For this review, take the finished solid that the model builds, in its own axes (mm). Give positions to 0.01 mm unless a question says otherwise; leave off trailing zeros. Loops run counter-clockwise (first coordinate to the right, second up) from the corner with the lowest first, then second, coordinate; pieces in that order, holes last. Notation, with made-up numbers: (51, 8.25) - (102, 8.25) arc R22 ccw to (102, 39.25) - close; hole circle Ø9 at (-17.5, 82.25). An arc over 180 degrees is marked (long way). Use CSV: the item, a comma, the result in double quotes. Start each with the question number.
1. Mouldability with a two-part tool opening along X and no side actions: class faces 1 (the cylindrical face through (2.71, 0.7, -62.203)), 2 (the flat face through (-50, -1, -222)), 3 (the flat face through (50, -1, -222)) as pulls with the +X half, pulls with the -X half, needs draft (parallel to the pull), parting line crosses it, or undercut.
2. Take a section at B-B on z = -50. Give the boundary of the cut face in (x, y), plus the area to 3 significant figures.
3. Wall thickness on line 1 (Z direction, x = 0, y = -3); line 2 (Z direction, x = -3.5, y = -14): over which ranges is each line inside the solid? List them lowest first.
4. For pin 1 (15 mm diameter, centred on x = 0, z = -50, fed in from +Y); pin 2 (5 mm diameter, centred on x = -18.5, y = -17.5, fed in from +Z), all flat-tipped, find the tip position at first contact; note any pin that passes through.
5. Take a section at A-A on x = 0. Give the boundary of the cut face in (y, z).
```python
from build123d import *

# Parameters (mm, degrees)
SKETCH2_W           = 100
SKETCH2_H           = 100
BOSS_EXTRUDE1_DEPTH = 450
SKETCH3_R           = 12.5
CUT_EXTRUDE1_DEPTH  = 500


with BuildPart() as part:
    # Sketch2 → Boss-Extrude1 (new body)
    with BuildSketch(Plane.XY):
        Rectangle(SKETCH2_W, SKETCH2_H)
    extrude(amount=-BOSS_EXTRUDE1_DEPTH)

    # Sketch3 → Cut-Extrude1 (cut)
    with BuildSketch(Plane(origin=(0, 50, 0), x_dir=(1, 0, 0), z_dir=(0, 1, 0))):
        with Locations(Location((0, 50, 0), (0, 0, 180))):
            Circle(SKETCH3_R)
    extrude(amount=-CUT_EXTRUDE1_DEPTH, mode=Mode.SUBTRACT)


solid = part.part
```
Check result:
1,face 1,"undercut"
1,face 2,"pulls with the -X half"
1,face 3,"pulls with the +X half"
2,outline,"(-50, -50) - (-12.5, -50) - (-12.5, 50) - (-50, 50) - close; (12.5, -50) - (50, -50) - (50, 50) - (12.5, 50) - close"
2,area,"7,500 mm²"
3,line 1,"z = -450 to -62.5, -37.5 to 0"
3,line 2,"z = -450 to -62, -38 to 0"
4,pin 1,"passes through"
4,pin 2,"stops at z = 0"
5,outline,"(-50, -450) - (50, -450) - (50, -62.5) - (-50, -62.5) - close; (-50, -37.5) - (50, -37.5) - (50, 0) - (-50, 0) - close"
